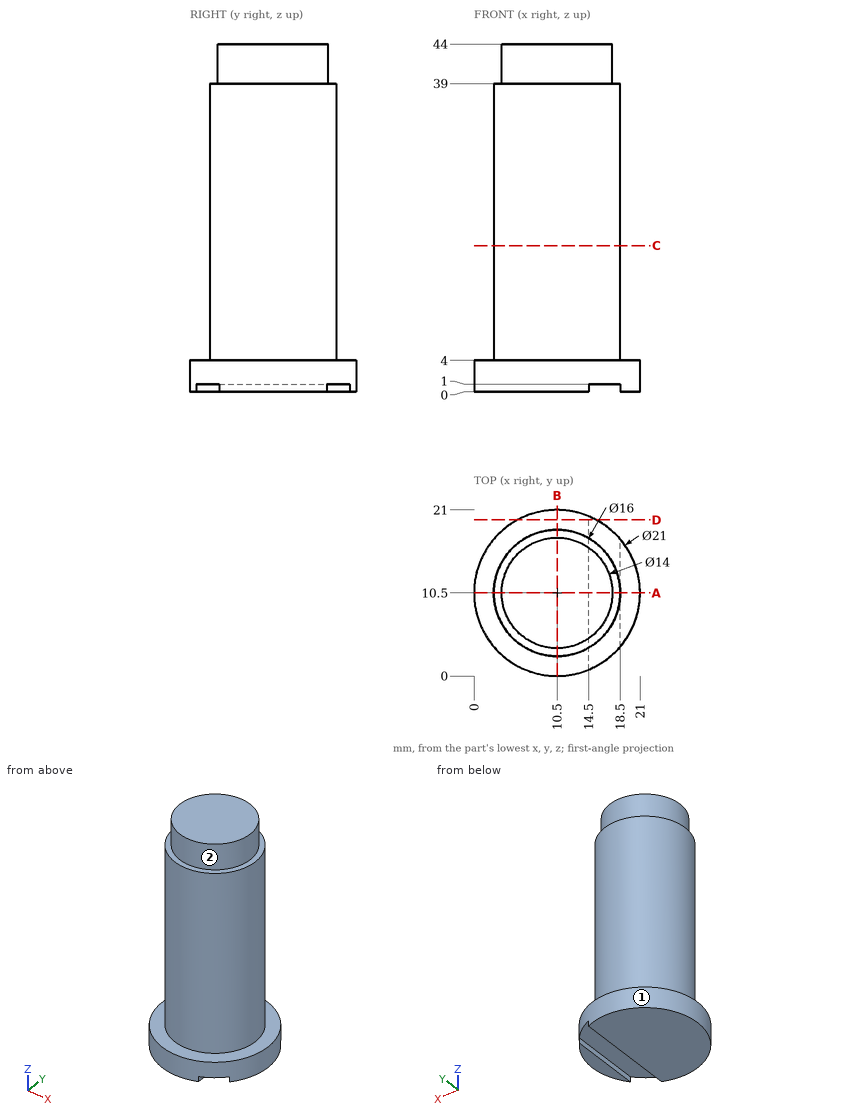
Geometry check sheet. Reference: drawing and pictorial views, mm from the part's lowest x, y, z. A direction names the side the tool comes from. Coordinates: 2 decimals unless noted, no trailing zeros. Order: outer loops, then holes, each group sorted by start corner. A loop starts at its lowest first (then second) coordinate and runs counter-clockwise, first axis right, second up.
Item 1: Section check B-B (x = 10.5). Enter the section's corners in (y, z).
Item 2: Tool access check on the marked faces 1 and 2. Record the directions out of +Z, -Z, +X, -X, +Y, -Y that give a thin tool (end or side, any length) a straight path to the whole face; none if there is none.
Item 3: Section check D-D (y = 19.75). Enter the section's corners in (x, z).
Item 4: Depth check by flat-ended pin: pin 1 (2 mm diameter, centred on x = 9.5, z = 33, fed in from +Y); pin 2 (5 mm diameter, centred on x = 8, z = 13.5, fed in from -Y); pin 3 (0.8 mm diameter, centred on y = 11.5, z = 0.5, fed in from -X); pin 4 (5 mm diameter, centred on x = 3, y = 6, fed in from +Z). Enter the tip coordinate at first touch or a pass-through.
Item 5: Section check C-C (z = 18.5). Enter the section's corners in (x, y), plus the area to 3 significant figures.
Item 6: Section check A-A (y = 10.5). Enter the section's corners in (x, z), plus the area to 3 significant figures.
Item 7: Scan lines: line 1 along Y through (x, z) = (10.75, 7.5); line 2 along Z through (x, y) = (17.5, 11.75); line 3 along Z through (x, y) = (16.5, 14). Record each from-to range of solid material in increasing order.
Check sheet entries:
1. outline: (0, 0) - (21, 0) - (21, 4) - (18.5, 4) - (18.5, 39) - (17.5, 39) - (17.5, 44) - (3.5, 44) - (3.5, 39) - (2.5, 39) - (2.5, 4) - (0, 4) - close
2. face 1: +Z, -Z
2. face 2: +Z
3. outline: (5.53, 0) - (14.5, 0) - (14.5, 1) - (15.47, 1) - (15.47, 4) - (5.53, 4) - close
4. pin 1: stops at y = 18.5
4. pin 2: stops at y = 2.5
4. pin 3: stops at x = 0.02
4. pin 4: stops at z = 44
5. outline: circle Ø16 at (10.5, 10.5)
5. area: 201 mm2
6. outline: (0, 0) - (14.5, 0) - (14.5, 1) - (18.5, 1) - (18.5, 0) - (21, 0) - (21, 4) - (18.5, 4) - (18.5, 39) - (17.5, 39) - (17.5, 44) - (3.5, 44) - (3.5, 39) - (2.5, 39) - (2.5, 4) - (0, 4) - close
6. area: 710 mm2
7. line 1: y = 2.5 to 18.5
7. line 2: z = 1 to 39
7. line 3: z = 1 to 44
